Can you work these out from the model? Positions are in its coordinate system, mm. A direction names the side the tool comes from. Round coordinates to 2 decimals unless told otherwise and drop trailing zeros. Loops run counter-clockwise (first coordinate to the right, second up) from the corner with the lowest first, then second, coordinate; pieces in that order, holes last. Notation, with made-up numbers: M 34,-23.75 L 53,-23.75 A25 cw 53,14.25 Z; hole C 13,33 d7. An arc over 180 degrees is marked long. Return JSON: item names as keys, results as strings.
```python
from build123d import *

# Parameters (mm, degrees)
F2_DEPTH = 90


with BuildPart() as f2:
    # F0 (on Top) → F2 (new body)
    with BuildSketch(Plane.XY):
        Polygon((0.75, 17.7535207776), (0, 17.3205080757), (15, 8.6602540378), (15, 9.5262794416), (15.75, 9.9592921435), (0.75, 18.6195461814), align=None)
        Polygon((-0.75, 17.7535207776), (0, 17.3205080757), (0.75, 17.7535207776), (0.75, 18.6195461814), (0, 19.0525588833), (-0.75, 18.6195461814), align=None)
        Polygon((-15, 8.6602540378), (0, 17.3205080757), (-0.75, 17.7535207776), (-0.75, 18.6195461814), (-15.75, 9.9592921435), (-16.5, 9.5262794416), (-16.5, 8.6602540378), (-15.75, 8.227241336), align=None)
        Polygon((15.75, 8.227241336), (15, 8.6602540378), (15, -8.6602540378), (15, -9.5262794416), (15.75, -9.9592921435), (16.5, -9.5262794416), (16.5, -8.6602540378), (16.5, 8.6602540378), align=None)
        Polygon((15, 9.5262794416), (15, 8.6602540378), (15.75, 8.227241336), (16.5, 8.6602540378), (16.5, 9.5262794416), (15.75, 9.9592921435), align=None)
        Polygon((-15, -8.6602540378), (-15, 8.6602540378), (-15.75, 8.227241336), (-16.5, 8.6602540378), (-16.5, -9.5262794416), (0, -19.0525588833), (15.75, -9.9592921435), (15, -9.5262794416), (15, -8.6602540378), (0, -17.3205080757), align=None)
        Polygon((0, 19.0525588833), (0.75, 18.6195461814), (0.75, 35.9400542571), (0, 35.5070415552), (-0.75, 35.9400542571), (-0.75, 18.6195461814), align=None)
        Polygon((30.75, 18.6195461814), (15.75, 9.9592921435), (16.5, 9.5262794416), (16.5, 8.6602540378), (31.5, 17.3205080757), (30.75, 17.7535207776), align=None)
        Polygon((-32.25, 17.7535207776), (-16.5, 8.6602540378), (-16.5, 9.5262794416), (-15.75, 9.9592921435), (-30.75, 18.6195461814), (-30.75, 35.9400542571), (-15.75, 44.6003082949), (-16.5, 45.0333209968), (-16.5, 45.8993464006), (-32.25, 36.8060796608), align=None)
        Polygon((0, 35.5070415552), (0.75, 35.9400542571), (0.75, 36.8060796608), (0, 37.2390923627), (-0.75, 36.8060796608), (-0.75, 35.9400542571), align=None)
        Polygon((0.75, 36.8060796608), (0.75, 35.9400542571), (15.75, 44.6003082949), (15, 45.0333209968), (15, 45.8993464006), (0, 37.2390923627), align=None)
        Polygon((-15.75, 44.6003082949), (-0.75, 35.9400542571), (-0.75, 36.8060796608), (0, 37.2390923627), (-15, 45.8993464006), (-15.75, 46.3323591025), (-16.5, 45.8993464006), (-16.5, 45.0333209968), align=None)
        Polygon((16.5, -9.5262794416), (15.75, -9.9592921435), (31.5, -19.0525588833), (47.25, -9.9592921435), (46.5, -9.5262794416), (46.5, -8.6602540378), (31.5, -17.3205080757), (16.5, -8.6602540378), align=None)
        Polygon((30.75, 35.9400542571), (30.75, 18.6195461814), (31.5, 19.0525588833), (32.25, 18.6195461814), (32.25, 35.9400542571), (31.5, 35.5070415552), align=None)
        Polygon((31.5, 19.0525588833), (30.75, 18.6195461814), (30.75, 17.7535207776), (31.5, 17.3205080757), (32.25, 17.7535207776), (32.25, 18.6195461814), align=None)
        Polygon((32.25, 17.7535207776), (31.5, 17.3205080757), (46.5, 8.6602540378), (46.5, 9.5262794416), (47.25, 9.9592921435), (32.25, 18.6195461814), align=None)
        Polygon((16.5, 45.0333209968), (15.75, 44.6003082949), (30.75, 35.9400542571), (30.75, 36.8060796608), (31.5, 37.2390923627), (16.5, 45.8993464006), align=None)
        Polygon((15, 45.0333209968), (15.75, 44.6003082949), (16.5, 45.0333209968), (16.5, 45.8993464006), (15.75, 46.3323591025), (15, 45.8993464006), align=None)
        Polygon((30.75, 36.8060796608), (30.75, 35.9400542571), (31.5, 35.5070415552), (32.25, 35.9400542571), (32.25, 36.8060796608), (31.5, 37.2390923627), align=None)
        Polygon((47.25, 8.227241336), (46.5, 8.6602540378), (46.5, -8.6602540378), (46.5, -9.5262794416), (47.25, -9.9592921435), (48, -9.5262794416), (48, -8.6602540378), (48, 8.6602540378), align=None)
        Polygon((46.5, 9.5262794416), (46.5, 8.6602540378), (47.25, 8.227241336), (48, 8.6602540378), (48, 9.5262794416), (47.25, 9.9592921435), align=None)
        Polygon((48, -9.5262794416), (47.25, -9.9592921435), (63, -19.0525588833), (79.5, -9.5262794416), (79.5, 8.6602540378), (78.75, 8.227241336), (78, 8.6602540378), (78, -8.6602540378), (63, -17.3205080757), (48, -8.6602540378), align=None)
        Polygon((-16.5, 64.08587988), (-16.5, 45.8993464006), (-15.75, 46.3323591025), (-15, 45.8993464006), (-15, 63.2198544763), (0, 71.8801085141), (15, 63.2198544763), (15, 64.08587988), (15.75, 64.5188925819), (0, 73.6121593217), align=None)
        Polygon((15, 63.2198544763), (15, 45.8993464006), (15.75, 46.3323591025), (16.5, 45.8993464006), (16.5, 63.2198544763), (16.5, 64.08587988), (15.75, 64.5188925819), (15, 64.08587988), align=None)
        Polygon((62.25, 18.6195461814), (47.25, 9.9592921435), (48, 9.5262794416), (48, 8.6602540378), (63, 17.3205080757), (62.25, 17.7535207776), align=None)
        Polygon((32.25, 36.8060796608), (32.25, 35.9400542571), (47.25, 44.6003082949), (46.5, 45.0333209968), (46.5, 45.8993464006), (31.5, 37.2390923627), align=None)
        Polygon((16.5, 64.08587988), (16.5, 63.2198544763), (31.5, 71.8801085141), (46.5, 63.2198544763), (46.5, 64.08587988), (47.25, 64.5188925819), (31.5, 73.6121593217), (15.75, 64.5188925819), align=None)
        Polygon((62.25, 35.9400542571), (62.25, 18.6195461814), (63, 19.0525588833), (63.75, 18.6195461814), (63.75, 35.9400542571), (63, 35.5070415552), align=None)
        Polygon((63, 19.0525588833), (62.25, 18.6195461814), (62.25, 17.7535207776), (63, 17.3205080757), (63.75, 17.7535207776), (63.75, 18.6195461814), align=None)
        Polygon((48, 45.0333209968), (47.25, 44.6003082949), (62.25, 35.9400542571), (62.25, 36.8060796608), (63, 37.2390923627), (48, 45.8993464006), align=None)
        Polygon((46.5, 45.0333209968), (47.25, 44.6003082949), (48, 45.0333209968), (48, 45.8993464006), (47.25, 46.3323591025), (46.5, 45.8993464006), align=None)
        Polygon((46.5, 63.2198544763), (46.5, 45.8993464006), (47.25, 46.3323591025), (48, 45.8993464006), (48, 63.2198544763), (48, 64.08587988), (47.25, 64.5188925819), (46.5, 64.08587988), align=None)
        Polygon((63.75, 17.7535207776), (63, 17.3205080757), (78, 8.6602540378), (78.75, 8.227241336), (79.5, 8.6602540378), (79.5, 9.5262794416), (78.75, 9.9592921435), (63.75, 18.6195461814), align=None)
        Polygon((79.5, 9.5262794416), (79.5, 8.6602540378), (95.25, 17.7535207776), (95.25, 36.8060796608), (79.5, 45.8993464006), (79.5, 45.0333209968), (78.75, 44.6003082949), (93.75, 35.9400542571), (93.75, 18.6195461814), (78.75, 9.9592921435), align=None)
        Polygon((62.25, 36.8060796608), (62.25, 35.9400542571), (63, 35.5070415552), (63.75, 35.9400542571), (63.75, 36.8060796608), (63, 37.2390923627), align=None)
        Polygon((63.75, 36.8060796608), (63.75, 35.9400542571), (78.75, 44.6003082949), (79.5, 45.0333209968), (79.5, 45.8993464006), (78.75, 46.3323591025), (78, 45.8993464006), (63, 37.2390923627), align=None)
        Polygon((48, 64.08587988), (48, 63.2198544763), (63, 71.8801085141), (78, 63.2198544763), (78, 45.8993464006), (78.75, 46.3323591025), (79.5, 45.8993464006), (79.5, 64.08587988), (63, 73.6121593217), (47.25, 64.5188925819), align=None)
    extrude(amount=F2_DEPTH)


solid = f2.part
```
Q1. If I drill on line 1 along X through (y, z) = (54, 8.5); line 2 along X through (y, z) = (26.5, 38); line 3 along Y through (x, z) = (7, 80), over which ranges is the centre line in solid material (lowest first)?
Results:
{"line 1": "x = -16.5 to -15, 15 to 16.5, 46.5 to 48, 78 to 79.5", "line 2": "x = -32.25 to -30.75, -0.75 to 0.75, 30.75 to 32.25, 62.25 to 63.75, 93.75 to 95.25", "line 3": "y = -15.01 to -13.28, 13.28 to 15.01, 39.55 to 41.28, 67.84 to 69.57"}
Q2. Suppose I cut it at C-C, the plane x = -24. Please give me the cut outline in (y, z).
Results:
{"outline": "M 12.99,0 L 14.72,0 L 14.72,90 L 12.99,90 Z; M 39.84,0 L 41.57,0 L 41.57,90 L 39.84,90 Z"}
Q3. Suppose I cut it at D-D, the plane y = -13. Please give me the cut outline in (x, z).
Results:
{"outline": "M -10.48,0 L -7.48,0 L -7.48,90 L -10.48,90 Z; M 7.48,0 L 10.48,0 L 10.48,90 L 7.48,90 Z; M 21.02,0 L 24.02,0 L 24.02,90 L 21.02,90 Z; M 38.98,0 L 41.98,0 L 41.98,90 L 38.98,90 Z; M 52.52,0 L 55.52,0 L 55.52,90 L 52.52,90 Z; M 70.48,0 L 73.48,0 L 73.48,90 L 70.48,90 Z"}
Q4. I'm going to push flat-ended pins straight in: pin 1 Ø14 at (y, z) = (54, 67.5) entering from -X; pin 2 Ø19 at (y, z) = (58, 46) entering from +X; pin 3 Ø10 at (x, z) = (40.5, 16.5) entering from -Y. Where does each tip first touch, or does it pass through?
Results:
{"pin 1": "stops at x = -16.5", "pin 2": "stops at x = 79.5", "pin 3": "stops at y = -16.74"}
Q5. On a 3-axis mill with a long thin cutter (end or side, diameter ignored), from which of +Z, -Z, +X, -X, +Y, -Y can I reach the whole of each face in a straight line? I mean faces 3 (the flat face through (39.49, 69, 44.37)), 4 (the flat face through (16.5, 0, 44)). Say none if no direction works.
Results:
{"face 3": "+Z, -Z, +Y", "face 4": "+Z, -Z"}
Q6. Suppose I cut it at A-A, the plane y = 0. Please give me the cut outline in (x, z).
Results:
{"outline": "M -16.5,0 L -15,0 L -15,90 L -16.5,90 Z; M 15,0 L 16.5,0 L 16.5,90 L 15,90 Z; M 46.5,0 L 48,0 L 48,90 L 46.5,90 Z; M 78,0 L 79.5,0 L 79.5,90 L 78,90 Z"}
Q7. Suppose I cut it at B-B, the plane y = 26. Please give me the cut outline in (x, z), plus the area to 3 significant figures.
Results:
{"outline": "M -32.25,0 L -30.75,0 L -30.75,90 L -32.25,90 Z; M -0.75,0 L 0.75,0 L 0.75,90 L -0.75,90 Z; M 30.75,0 L 32.25,0 L 32.25,90 L 30.75,90 Z; M 62.25,0 L 63.75,0 L 63.75,90 L 62.25,90 Z; M 93.75,0 L 95.25,0 L 95.25,90 L 93.75,90 Z", "area": "675 mm2"}
Q8. Thinking about a two-plate mould opening in X: for faces 1 (the flat face through (-7.605, 12.93, 44.37)), 2 (the flat face through (31, 27, 0)), which applies, pulls with the +X half, pulls with the -X half, needs draft (parallel to the pull), parting line crosses it, or undercut?
Results:
{"face 1": "undercut", "face 2": "needs draft"}
